Geometry: final body of the model. Coordinates: model frame, mm. Face numbers are marked on the shaded views. A direction names the side the tool comes from. Coordinates: 2 decimals unless noted, no trailing zeros. Order: outer loops, then holes, each group sorted by start corner. A loop starts at its lowest first (then second) coordinate and runs counter-clockwise, first axis right, second up. Notation, with made-up numbers: (78.25, -18.75) -> (129.25, -18.75) arc R19 ccw to (129.25, -10.75) -> close; hole circle Ø7 at (-19, 18). An arc over 180 degrees is marked (long way). Use one line per item in the form item = value.
```python
from build123d import *

# Parameters (mm, degrees)
SKETCH3_W           = 7.8
SKETCH3_H           = 3.175
SKETCH3_W_2         = 31.75
BOSS_EXTRUDE2_DEPTH = 63.5
SKETCH4_R           = 4.365625
SKETCH4_R_2         = 1.7
CUT_EXTRUDE1_DEPTH  = 7.35
FILLET1_R           = 1.5875


with BuildPart() as part:
    # Sketch3 → Boss-Extrude2 (new body)
    with BuildSketch(Plane.XY):
        with Locations((15.875, -1.5875)):
            Rectangle(SKETCH3_W, SKETCH3_H)
        with Locations((15.875, 1.5875)):
            Rectangle(SKETCH3_W_2, SKETCH3_H)
    extrude(amount=BOSS_EXTRUDE2_DEPTH)

    # Sketch4 → Cut-Extrude1 (cut, through all)
    with BuildSketch(Plane(origin=(0, 3.175, 0), x_dir=(1, 0, 0), z_dir=(0, 1, 0))):
        with BuildLine():
            Line((10, -49.1), (31.75, -49.1))
            Line((31.75, -49.1), (31.75, -33.45))
            Line((31.75, -33.45), (10, -33.45))
            ThreePointArc((10, -33.45), (8.232233047, -34.182233047), (7.5, -35.95))
            Line((7.5, -35.95), (7.5, -46.6))
            ThreePointArc((7.5, -46.6), (8.232233047, -48.367766953), (10, -49.1))
        make_face()
        with Locations((15.875, -9.525)):
            Circle(SKETCH4_R)
        with Locations((15.875, -25.4)):
            Circle(SKETCH4_R_2)
        with Locations((15.875, -57.15)):
            Circle(SKETCH4_R_2)
    extrude(amount=-CUT_EXTRUDE1_DEPTH, mode=Mode.SUBTRACT)

    # Fillet1
    fillet1_edges = [part.edges().sort_by_distance(p)[0] for p in [
        (0, 1.5875, 0),
        (31.75, 1.5875, 0),
        (31.75, 1.5875, 63.5),
        (0, 1.5875, 63.5),
        (31.75, 1.5875, 33.45),
        (31.75, 1.5875, 49.1),
    ]]
    fillet(fillet1_edges, radius=FILLET1_R)


solid = part.part
```
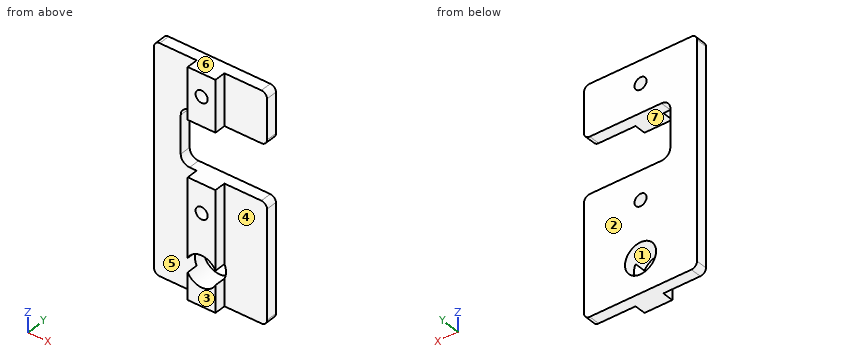
1) Material intervals for probe 1 along Z at (x, y) = (30, 1.75); probe 2 along Z at (x, y) = (15, -1.75); probe 3 along X at (y, z) = (-0.75, 25.4) (3 decimals), sorted ascending. Write a range as from..to.
Results found:
probe_1 = 0..33.45, 49.1..63.5
probe_2 = 0..5.25, 13.8..23.94, 26.86..33.45, 49.1..55.69, 58.61..63.5
probe_3 = 11.975..14.175, 17.575..19.775
2) Section B-B, the plane y = -0.75. Output: boundary loops of the cut face in (x, z) (3 decimals), and give its area (3 significant figures).
Results found:
outline = (11.975, 0) -> (19.775, 0) -> (19.775, 7.563) arc R4.366 cw to (11.975, 7.563) -> close; (11.975, 11.487) arc R4.366 cw to (19.775, 11.487) -> (19.775, 33.45) -> (11.975, 33.45) -> close; (11.975, 49.1) -> (19.775, 49.1) -> (19.775, 63.5) -> (11.975, 63.5) -> close; hole circle Ø3.4 at (15.875, 25.4); hole circle Ø3.4 at (15.875, 57.15)
area = 298 mm2
3) Pull-direction query (X, two-part tool) for the marked faces 1 and 2; classes: released by +X, released by -X, zero draft, split by the parting line, or undercut.
Results found:
face_1 = undercut
face_2 = zero draft
4) Contact query for flat-ended pins moving along their axis: P1, Ø1, axis at y = -2.5, z = 55, coming from the -X side (3 decimals); P2, Ø2.5, axis at y = -2, z = 57.5, coming from the +X side (3 decimals); P3, Ø3.5, axis at x = 24.5, z = 16, coming from the -Y side; P4, Ø3, axis at x = 15.875, z = 57.15, coming from the -Y side. Output: stop coordinate, or through.
Results found:
P1 = 11.975
P2 = 19.775
P3 = 0
P4 = through
5) Section D-D, the plane y = 2.5. Give the number of separate pieces and of enclosed holes in the cut face, and give its area (3 significant figures).
Results found:
separate_pieces = 1
enclosed_holes = 3
area = 1,560 mm2
6) Section A-A, the plane z = 57.15. Output: boundary loops of the cut face in (x, y) (3 decimals), and give its area (3 significant figures).
Results found:
outline = (0, 0) -> (11.975, 0) -> (11.975, -3.175) -> (14.175, -3.175) -> (14.175, 3.175) -> (0, 3.175) -> close; (17.575, -3.175) -> (19.775, -3.175) -> (19.775, 0) -> (31.75, 0) -> (31.75, 3.175) -> (17.575, 3.175) -> close
area = 104 mm2
7) Section C-C, the plane x = 23. Output: boundary loops of the cut face in (y, z) (3 decimals).
Results found:
outline = (0, 0) -> (3.175, 0) -> (3.175, 33.45) -> (0, 33.45) -> close; (0, 49.1) -> (3.175, 49.1) -> (3.175, 63.5) -> (0, 63.5) -> close
8) Access query for the marked faces 3, 4, 5, 6 and 7. Directions: +Z, -Z, +X, -X, +Y, -Y. A direction counts if a zero-diameter tool reaches every point of the face in a straight line with its end or side. Return the directions, or none.
Results found:
face_3 = +Z, -Z, +X, -X, -Y
face_4 = +Z, -Z, +X, -Y
face_5 = +Z, -Z, -X, -Y
face_6 = +Z, +X, -X, +Y, -Y
face_7 = +X, +Y, -Y
